```python
from build123d import *

# Parameters (mm, degrees)
SKETCH1_W           = 25.4
SKETCH1_H           = 76.2
BOSS_EXTRUDE1_DEPTH = 19.05
SKETCH2_R           = 31.75
CUT_EXTRUDE1_DEPTH  = 25.4
SKETCH4_W           = 7.62
SKETCH4_H           = 38.1
CUT_EXTRUDE3_DEPTH  = 26.4


with BuildPart() as part:
    # Sketch1 → Boss-Extrude1 (new body)
    with BuildSketch(Plane.XY):
        with Locations((12.7, 38.1)):
            Rectangle(SKETCH1_W, SKETCH1_H)
    extrude(amount=BOSS_EXTRUDE1_DEPTH)

    # Sketch2 → Cut-Extrude1 (cut)
    with BuildSketch(Plane.XY.offset(19.05)):
        with Locations((-12.7, 38.1)):
            Circle(SKETCH2_R)
    extrude(amount=-CUT_EXTRUDE1_DEPTH, mode=Mode.SUBTRACT)

    # Sketch4 → Cut-Extrude3 (cut, through all)
    with BuildSketch(Plane(origin=(25.4, 0, 0), x_dir=(0, 0, -1), z_dir=(1, 0, 0))):
        with Locations((-15.24, 38.1)):
            Rectangle(SKETCH4_W, SKETCH4_H)
    extrude(amount=-CUT_EXTRUDE3_DEPTH, mode=Mode.SUBTRACT)


solid = part.part
```
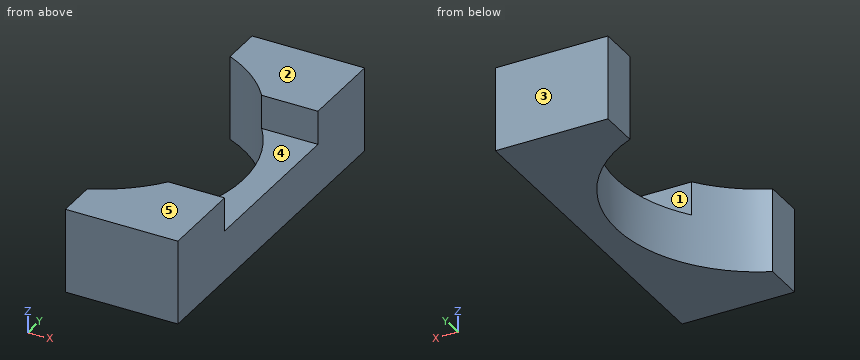
Could you check a few things on this model? Use its own coordinates, in mm. Face numbers are marked on the shaded views. A direction names the side the tool comes from. Round coordinates to 2 decimals unless told otherwise and drop trailing zeros. Order: outer loops, then holes, each group sorted by start corner. A loop starts at its lowest first (then second) coordinate and runs counter-clockwise, first axis right, second up. Notation, with made-up numbers: (26.25, 27.25) -> (67.25, 27.25) arc R17 ccw to (67.25, 53.25) -> close; hole circle Ø9 at (10.25, 64.5). An arc over 180 degrees is marked (long way). One line per question, with ' | ' between items.
Q1. Which directions (+Z, -Z, +X, -X, +Y, -Y) give clear straight access to the entire face, cutting with the end or side of a thin tool? Please do the marked faces 4 and 5.
Computed values:
face 4: +Z, +X, -X | face 5: +Z, +X, -X, +Y, -Y
Q2. If I drill on line 1 (Y direction, x = 14.25, z = 17.5); line 2 (Z direction, x = 20.75, y = 24); line 3 (Y direction, x = 6.5, z = 10), over which ranges is the centre line in solid material (lowest first)? Write a range as from..to.
Computed values:
line 1: 0..19.05, 57.15..76.2 | line 2: 0..11.43 | line 3: 0..12.81, 63.39..76.2
Q3. If we section it at B-B on x = 4.5: Write out the boundary of the cut face in (y, z), plus the area to 3 significant figures.
Computed values:
outline: (0, 0) -> (11.41, 0) -> (11.41, 19.05) -> (0, 19.05) -> close; (64.79, 0) -> (76.2, 0) -> (76.2, 19.05) -> (64.79, 19.05) -> close | area: 435 mm²
Q4. If we section it at C-C on z = 10.25: Write out the boundary of the cut face in (x, y).
Computed values:
outline: (0, 0) -> (25.4, 0) -> (25.4, 76.2) -> (0, 76.2) -> (0, 67.2) arc R31.75 cw to (0, 9) -> close
Q5. We'd pull the mould along Y, two halves only. Please class the marked faces 1, 2 and 3: released by +Y, released by -Y, zero draft, split by the parting line, or undercut.
Computed values:
face 1: undercut | face 2: zero draft | face 3: released by +Y
Q6. If we section it at D-D on x = 11.5: Write out the boundary of the cut face in (y, z).
Computed values:
outline: (0, 0) -> (17.55, 0) -> (17.55, 19.05) -> (0, 19.05) -> close; (58.65, 0) -> (76.2, 0) -> (76.2, 19.05) -> (58.65, 19.05) -> close
Q7. If we section it at A-A on z = 14.25: Write out the boundary of the cut face in (x, y).
Computed values:
outline: (0, 0) -> (25.4, 0) -> (25.4, 19.05) -> (12.7, 19.05) arc R31.75 cw to (0, 9) -> close; (0, 67.2) arc R31.75 cw to (12.7, 57.15) -> (25.4, 57.15) -> (25.4, 76.2) -> (0, 76.2) -> close
Q8. I'm going to push flat-ended pins straight in: pin 1 (3 mm diameter, centred on x = 20, y = 23.5, fed in from +Z); pin 2 (8 mm diameter, centred on x = 9, y = 51, fed in from +Z). Where does each tip first touch, or does it pass through?
Computed values:
pin 1: z = 11.43 | pin 2: through
